Autodesk Inventor part; units mm, degrees
ref_plane "YZ Plane" through (0, 0, 0) normal (1, 0, 0) x (0, 1, 0)
ref_plane "XZ Plane" through (0, 0, 0) normal (0, 1, 0) x (-1, 0, 0)
ref_plane "XY Plane" through (0, 0, 0) normal (0, 0, 1) x (1, 0, 0)
sketch "Sketch1" plane through (0, 0, 0) normal (0, 0, 1) x (1, 0, 0)
  circle A0 centre (0, 0) radius 14.5
  dimension "d0" = 29
extrude "Extrusion1" add sketch "Sketch1" along normal blind 86
sketch "Sketch2" plane through (0, 0, 0) normal (0, 0, -1) x (-1, 0, 0)
  circle A0 centre (0, 0) radius 14.5
  circle A1 centre (0, 0) radius 7.5
  dimension "d3" = 15
extrude "Extrusion2" cut sketch "Sketch2" against normal blind 10
sketch "Sketch3" plane through (0, 0, 0) normal (0, 0, -1) x (-1, 0, 0)
  circle A0 centre (0, 0) radius 3.5
  dimension "d6" = 7
extrude "Extrusion3" cut sketch "Sketch3" against normal blind 10
properties part number "motor29x86"
The listing builds one solid part. Answer for the finished solid, in the listing's coordinates (mm). A direction names the side the tool comes from. Give positions to 0.01 mm unless a question says otherwise; leave off trailing zeros. Write each loop counter-clockwise with the first axis right and the second up, starting at its lowest first coordinate (ties: lowest second). Pieces come first, ordered by that corner, then holes.
Item 1: Which of the six approach directions +Z, -Z, +X, -X, +Y, -Y give full straight-line access (tool end or side, diameter ignored) to faces 4 (the cylindrical face through (6.691, 12.864, 47.468)), 5 (the flat face through (0, 0, 10))?
Item 2: Section D-D, the plane z = 58 is taken. Write down the section's boundary in (x, y).
Item 3: Section A-A, the plane x = 0 is taken. Write down the section's boundary in (y, z).
Item 4: Flat-ended cylindrical pins translate along their axes: P1, Ø12, axis at x = -0.5, z = 33, coming from the -Y side; P2, Ø2, axis at x = 6, y = 8, coming from the -Z side; P3, Ø2, axis at y = -4.5, z = 10, coming from the -X side; P4, Ø6, axis at x = -4.5, z = 72, coming from the -Y side. Find the tip coordinate at first contact, or state that the pin passes through.
Item 5: Find the intervals of material crossed by line 1 along Y through (x, z) = (0, 3.5); line 2 along Z through (x, y) = (2, -13); line 3 along Y through (x, z) = (-0.25, 12), in increasing order.
Item 6: Determine the mould class of faces 1 (the cylindrical face through (7.493, 0.33, 4.93)), 2 (the cylindrical face through (-3.233, -1.341, 4.93)), 3 (the flat face through (3.2, 1.8, 0)) for opening direction Y: released by +Y, released by -Y, zero draft, split by the parting line, or undercut.
Item 7: Section C-C, the plane z = 8 is taken. Write down the section's boundary in (x, y), plus the area to 3 significant figures.
Completed:
1. face 4: +Z, -Z
1. face 5: -Z
2. outline: circle Ø29 at (0, 0)
3. outline: (-14.5, 10) - (-7.5, 10) - (-7.5, 0) - (-3.5, 0) - (-3.5, 10) - (3.5, 10) - (3.5, 0) - (7.5, 0) - (7.5, 10) - (14.5, 10) - (14.5, 86) - (-14.5, 86) - close
4. P1: stops at y = -14.5
4. P2: stops at z = 10
4. P3: stops at x = -14.07
4. P4: stops at y = -14.42
5. line 1: y = -7.5 to -3.5, 3.5 to 7.5
5. line 2: z = 10 to 86
5. line 3: y = -14.5 to 14.5
6. face 1: split by the parting line
6. face 2: undercut
6. face 3: zero draft
7. outline: circle Ø15 at (0, 0); hole circle Ø7 at (0, 0)
7. area: 138 mm2
